Autodesk Inventor part; units mm, degrees
ref_plane "YZ Plane" through (0, 0, 0) normal (1, 0, 0) x (0, 1, 0)
ref_plane "XZ Plane" through (0, 0, 0) normal (0, 1, 0) x (-1, 0, 0)
ref_plane "XY Plane" through (0, 0, 0) normal (0, 0, 1) x (1, 0, 0)
sketch "Szkic1" plane through (0, 0, 0) normal (0, 0, 1) x (1, 0, 0)
  line L0 (-43.0447, 20.476) -> (-43.0447, -18.4903)
  line L1 (22.9553, 20.2216) -> (22.9553, -18.4903)
  line L2 (-21.0447, 5.0097) -> (-21.0447, -9.9903)
  line L3 (0.9553, 5.0097) -> (0.9553, -9.9903)
  line L4 (-43.0447, -18.4903) -> (22.9553, -18.4903)
  line L5 (-43.0447, -9.9903) -> (-21.0447, -9.9903)
  line L6 (0.9553, -9.9903) -> (22.9553, -9.9903)
  line L7 (-21.0447, 5.0097) -> (0.9553, 5.0097)
  line L8 (-21.0447, 5.0097) -> (-43.0447, 11.1338)
  line L9 (-10.2095, 11.3357) -> (-43.0447, 20.476)
  line L10 (0.9553, 5.0097) -> (22.9553, 10.9042)
  line L11 (-10.2095, 11.3357) -> (22.9553, 20.2216)
  point P0 (0, 0)
  point P1 (-37.0447, -14.4903)
  point P2 (16.955, -14.6697)
  point P3 (-37.0447, 14.1347)
  point P4 (16.9553, 13.9553)
  dimension "d0" = 66
  dimension "d1" = 54
  dimension "d2" = 6
  dimension "d3" = 54
  dimension "d4" = 6
  dimension "d5" = 28.625
  dimension "d6" = 22
  dimension "d7" = 22
  dimension "d8" = 4
  dimension "d10" = 23.5
  dimension "d11" = 4.5
  dimension "d12" = 9
  dimension "d13" = 28.625
  dimension "d14" = 4.5
  dimension "d15" = 9
extrude "Wyciągnięcie proste1" add sketch "Szkic1" along normal blind 4.5 contours L9 L11 L1 L10 L7 L8 L0 | L5 L2 L7 L3 L6 L1 L4 L0
hole "Otwór1" at (-37.0447, -14.4903, 0) at (16.955, -14.6697, 0) at (-37.0447, 14.1347, 0) at (16.9553, 13.9553, 0) direction (0, 0, 1) diameter 3.25 end through all
sketch "Szkic2" plane through (0, 0, 4.5) normal (0, 0, 1) x (1, 0, 0)
  line L0 (-21.0447, 5.0097) -> (-21.0447, -9.9903)
  line L1 (-21.0447, 5.0097) -> (0.7211, 5.0097)
  circle A0 centre (-37.0447, 14.1347) radius 1.625
  circle A1 centre (-37.0447, -14.4903) radius 1.625
  circle A2 centre (16.955, -14.6697) radius 1.625
  circle A3 centre (16.9553, 13.9553) radius 1.625
  line L2 (-43.0447, 20.476) -> (-43.0447, 11.1338)
  line L3 (-43.0447, 11.1338) -> (-21.0447, 5.0097)
  line L4 (-21.0447, 5.0097) -> (-21.0447, -9.9903)
  line L5 (-21.0447, -9.9903) -> (-43.0447, -9.9903)
  line L6 (-43.0447, -9.9903) -> (-43.0447, -18.4903)
  line L7 (-43.0447, -18.4903) -> (22.9553, -18.4903)
  line L8 (22.9553, -18.4903) -> (22.9553, -9.9903)
  line L9 (22.9553, -9.9903) -> (0.9553, -9.9903)
  line L10 (0.9553, -9.9903) -> (0.9553, 5.0097)
  line L11 (0.9553, 5.0097) -> (22.9553, 10.9042)
  line L12 (22.9553, 10.9042) -> (22.9553, 20.2216)
  line L13 (22.9553, 20.2216) -> (-10.2095, 11.3357)
  line L14 (-10.2095, 11.3357) -> (-43.0447, 20.476)
  line L15 (-21.0447, -4.9903) -> (0.9553, -4.9903)
  line L16 (-43.0447, -18.4903) -> (22.9553, -18.4903)
  line L17 (-21.0447, -4.9903) -> (0.9553, -4.9903)
  line L18 (0.9553, -4.9903) -> (0.9553, -18.4903)
  line L19 (0.9553, -18.4903) -> (-21.0447, -18.4903)
  line L20 (-21.0447, -18.4903) -> (-21.0447, -4.9903)
  line L21 (-21.0447, 5.0097) -> (0.9553, 5.0097)
  line L22 (0.9553, 5.0097) -> (0.9553, -4.9903)
  line L23 (0.9553, -4.9903) -> (-21.0447, -4.9903)
  line L24 (-21.0447, -4.9903) -> (-21.0447, 5.0097)
  circle A4 centre (-37.0447, 14.1347) radius 3.1
  circle A5 centre (16.9553, 13.9553) radius 3.1
  circle A6 centre (16.955, -14.6697) radius 3.1
  circle A7 centre (-37.0447, -14.4903) radius 3.1
  point P0 (0, 0)
  dimension "d25" = 13.5
  dimension "d31" = 6.2
  dimension "d32" = 6.2
  dimension "d33" = 6.2
  dimension "d34" = 6.2
extrude "Wyciągnięcie proste2" add sketch "Szkic2" along normal blind 11 contours L15 L10 L18 L7 L20 L0
extrude "Wyciągnięcie proste3" add sketch "Szkic2" along normal blind 23 contours L1 L21 L10 L15 L0
fillet "Zaokrąglenie1" radius 4 11 edges at (22.9553, 10.9042, 2.25) (22.9553, 20.2216, 2.25) (-10.2095, 11.3357, 2.25) (-43.0447, 20.476, 2.25) (-43.0447, 11.1338, 2.25) (0.9553, -9.9903, 2.25) (22.9553, -9.9903, 2.25) (22.9553, -18.4903, 2.25) (-43.0447, -18.4903, 2.25) (-43.0447, -9.9903, 2.25) (-21.0447, -9.9903, 2.25)
extrude "Wyciągnięcie proste4" cut sketch "Szkic2" against normal blind 2 contours A4 | A5 | A6 | A7
fillet "Zaokrąglenie2" radius 3 3 edges at (-10.0447, 5.0097, 4.5) (-21.0447, -12.2403, 4.5) (0.9553, -12.2403, 4.5)
fillet "Zaokrąglenie3" radius 2.5 2 edges at (-21.0447, 0.0097, 27.5) (0.9553, 0.0097, 27.5)
sketch "Szkic3" plane through (-21.0447, -18.4903, 15.5) normal (0, -1, 0) x (1, 0, 0)
  line L0 (22, 0) -> (0, 0)
  line L1 (0, -8) -> (0, 0)
  arc A0 (2.925, 0) -> (19.075, 0) centre (11, 0) ccw
  arc A1 (4.95, 0) -> (17.05, 0) centre (11, 0) ccw
  point P0 (21.0447, -15.5)
  dimension "d39" = 11
  dimension "d48" = 16.15
  dimension "d51" = 12.1
hole "Otwór2" at (-10.0447, -18.4903, 15.5) direction (0, 1, 0) diameter 4.2 end through all
extrude "Wyciągnięcie proste5" cut sketch "Szkic3" against normal blind 12.9
extrude "Wyciągnięcie proste6" add sketch "Szkic3" against normal blind 8.55 contours A0 L0 A1
extrude "Wyciągnięcie proste7" cut sketch "Szkic3" against normal blind 3.45 contours A0 L0 A1
sketch "Szkic4" plane through (0, 0, 15.5) normal (0, 0, 1) x (1, 0, 0)
  line L0 (-3.9947, -15.0403) -> (-1.9697, -15.0403)
  line L1 (-3.9947, -9.9403) -> (-1.9697, -9.9403)
  line L2 (0.9553, -18.4903) -> (0.9553, -4.9903)
  line L3 (-3.9947, -15.0403) -> (-3.9947, -9.9403)
  line L4 (-18.1197, -9.9403) -> (-16.0947, -9.9403)
  line L5 (-21.0447, -4.9903) -> (-21.0447, -18.4903)
  point P0 (0, 0)
  point P1 (-18.5697, -12.4903)
  point P2 (-1.5197, -12.4903)
  dimension "d56" = 5.1
  dimension "d57" = 4.95
  dimension "d58" = 2.475
  dimension "d59" = 2.55
  dimension "d60" = 2.55
  dimension "d61" = 2.475
hole "Otwór3" at (-18.5697, -12.4903, 15.5) at (-1.5197, -12.4903, 15.5) direction (0, 0, -1) diameter 3.2 end through all
sketch "Szkic5" plane through (0, 0, 0) normal (0, 0, -1) x (-1, 0, 0)
  circle A0 centre (18.5697, -12.4903) radius 1.6
  circle A1 centre (1.5197, -12.4903) radius 1.6
  circle A2 centre (18.5697, -12.4903) radius 3.1
  circle A3 centre (1.5197, -12.4903) radius 3.1
  point P0 (0, 0)
  dimension "d69" = 6.2
  dimension "d70" = 6.2
extrude "Wyciągnięcie proste8" cut sketch "Szkic5" against normal blind 3
sketch "Szkic6" plane through (-21.0447, -5.5903, 15.5) normal (0, -1, 0) x (1, 0, 0)
  arc A0 (7, 0) -> (15, 0) centre (11, 0) ccw
  line L0 (7, 0) -> (7, 8.5)
  line L1 (8.5, 10) -> (13.5, 10)
  line L2 (15, 8.5) -> (15, 0)
  arc A1 (8.9, 0) -> (13.1, 0) centre (11, 0) ccw
  arc A2 (8.5, 10) -> (7, 8.5) centre (8.5, 8.5) ccw
  arc A3 (15, 8.5) -> (13.5, 10) centre (13.5, 8.5) ccw
  point P0 (21.0447, -15.5)
  point P1 (7, 10)
  dimension "d73" = 8
  dimension "d74" = 10
  dimension "d75" = 1.5
extrude "Wyciągnięcie proste9" cut sketch "Szkic6" against normal blind 1.8
chamfer "Faza1" distance 0.5 angle 45 2 edges at (-10.0447, 5.0097, 17.6) (-10.0447, -3.7903, 17.6)
equation "\"d9\" = d8"
properties part number "3DP_ABS_E3DV6_Mount"
Design review of the part built by this model. Coordinates are the model's own, in mm. A direction names the side the tool comes from. Round coordinates to 2 decimals unless told otherwise and drop trailing zeros. Write each loop counter-clockwise with the first axis right and the second up, starting at its lowest first coordinate (ties: lowest second). Pieces come first, ordered by that corner, then holes. Notation, with made-up numbers: (59, -6.75) - (88, -6.75) arc R25 ccw to (88, 13.25) - close; hole circle Ø8 at (73, 45.25). An arc over 180 degrees is marked (long way). Use a Markdown table: item, result. Add a question column.
1. We need section D-D (y = -7.5). State the section outline as (x, z) points (3 decimals), then the cut area to 3 significant figures.
2. Mouldability with a two-part tool opening along X and no side actions: class faces 1 (the face through (-1, -10, 15.5)), 2 (the face through (0.2, 0.08, 26.79)), 3 (the face through (-10, -5.59, 11)) as +X half, -X half, draft (parallel to the pull), parting line (faces both ways), or undercut.
3. For faces 4 (the face through (10.34, 7.524, 2.864)), 5 (the face through (-32, -9.99, 2)), 6 (the face through (-24.43, 15.294, 2.218)), 7 (the face through (-11, 11, 4.5)), list the 3-axis set-ups (+Z, -Z, +X, -X, +Y, -Y) from which the entire face can be reached by the end or side of a thin tool; tool diameter is ignored.
4. We need section A-A (z = 23). State the section outline as (x, y) points, then the cut area to 3 significant figures.
5. We need section B-B (x = -26). State the section outline as (y, z) points.
6. Wall thickness on probe 1 along X at (y, z) = (-12.5, 12.5); probe 2 along Z at (x, y) = (-34.5, -10.5); probe 3 along Y at (x, z) = (-0.5, 12.5): over which ranges is each line inside the solid? List them lowest first.
7. Clearance check with flat-ended pins moving along their axes: pin 1 (1 mm diameter, centred on x = -3.5, z = 19.5, fed in from +Y); pin 2 (7 mm diameter, centred on x = -36, y = -15.5, fed in from +Z); pin 3 (5.5 mm diameter, centred on x = 16.95, y = -14.67, fed in from -Z); pin 4 (1.9 mm diameter, centred on x = -1.5, y = -14, fed in from -Z). State where each tip first meets the part, or that it passes through.
8. We need section C-C (y = 2). State the section outline as (x, z) points, then the cut area to 3 significant figures.
Output:
| question | item | result |
|---|---|---|
| 1 | outline | (-21.341, 0) - (1.251, 0) - (1.251, 6.201) arc R3 cw to (0.955, 7.5) - (0.955, 15.5) - (-1.97, 15.5) arc R8.075 cw to (-18.12, 15.5) - (-21.045, 15.5) - (-21.045, 7.5) arc R3 cw to (-21.341, 6.201) - close |
| 1 | area | 242 mm2 |
| 2 | face 1 | draft |
| 2 | face 2 | +X half |
| 2 | face 3 | undercut |
| 3 | face 4 | +Z, -Z, +X |
| 3 | face 5 | +Z, -Z, -X |
| 3 | face 6 | +Z, -Z, +Y |
| 3 | face 7 | +Z, +X, -X, +Y |
| 4 | outline | (-21.04, -4.99) - (-14.04, -4.99) - (-14.04, -3.79) - (-6.04, -3.79) - (-6.04, -4.99) - (0.96, -4.99) - (0.96, 5.01) - (-21.04, 5.01) - close |
| 4 | area | 210 mm2 |
| 5 | outline | (-18.49, 0) - (-9.99, 0) - (-9.99, 4.5) - (-18.49, 4.5) - close; (6.39, 0) - (15.73, 0) - (15.73, 4.5) - (8.01, 4.5) arc R3 cw to (6.39, 4.98) - close |
| 6 | probe 1 | x = -21.04 to -20.17, -16.97 to -15.3, -4.79 to -3.12, 0.08 to 0.96 |
| 6 | probe 2 | z = 0 to 4.5 |
| 6 | probe 3 | y = -18.49 to -13.72, -11.26 to 5.01 |
| 7 | pin 1 | stops at y = 5.01 |
| 7 | pin 2 | stops at z = 4.5 |
| 7 | pin 3 | stops at z = 0 |
| 7 | pin 4 | stops at z = 3 |
| 8 | outline | (-21.04, 0) - (0.96, 0) - (0.96, 25) arc R2.5 ccw to (-1.54, 27.5) - (-18.54, 27.5) arc R2.5 ccw to (-21.04, 25) - close; hole circle Ø4.2 at (-10.04, 15.5) |
| 8 | area | 588 mm2 |
